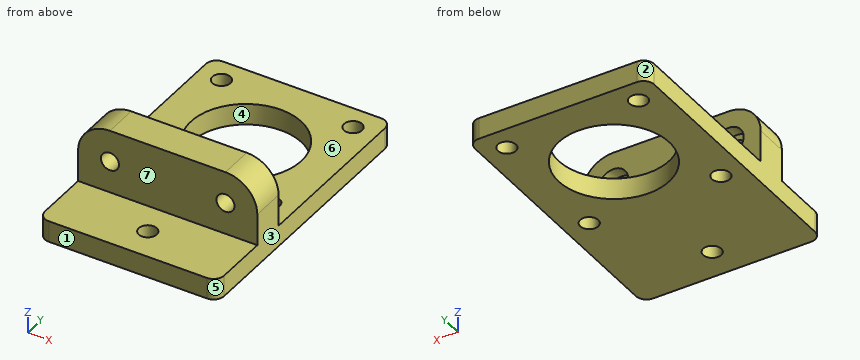
```python
from build123d import *

# Parameters (mm, degrees)
F0_R     = 2.125
F0_R_2   = 13
F1_DEPTH = 5
F2_W     = 42.2
F2_H     = 8
F3_DEPTH = 15
F4_R     = 7.5
F5_R     = 2.125
F6_DEPTH = 23.001
F7_R     = 3.5
F8_DEPTH = 3


with BuildPart() as f1:
    # F0 (on Top) → F1 (new body)
    with BuildSketch(Plane.XY):
        with BuildLine():
            Line((18.6, 21.1), (-18.6, 21.1))
            ThreePointArc((-18.6, 21.1), (-20.367767, 20.367767), (-21.1, 18.6))
            Line((-21.1, 18.6), (-21.1, -42))
            ThreePointArc((-21.1, -42), (-20.367767, -43.767767), (-18.6, -44.5))
            Line((-18.6, -44.5), (18.6, -44.5))
            ThreePointArc((18.6, -44.5), (20.367767, -43.767767), (21.1, -42))
            Line((21.1, -42), (21.1, 18.6))
            ThreePointArc((21.1, 18.6), (20.367767, 20.367767), (18.6, 21.1))
        make_face()
        with Locations((-15.5, -15.5)):
            Circle(F0_R, mode=Mode.SUBTRACT)
        with Locations((0, -37)):
            Circle(F0_R, mode=Mode.SUBTRACT)
        with Locations((15.5, -15.5)):
            Circle(F0_R, mode=Mode.SUBTRACT)
        with Locations((-15.5, 15.5)):
            Circle(F0_R, mode=Mode.SUBTRACT)
        Circle(F0_R_2, mode=Mode.SUBTRACT)
        with Locations((15.5, 15.5)):
            Circle(F0_R, mode=Mode.SUBTRACT)
    extrude(amount=F1_DEPTH)

    # F2 (on face) → F3 (join)
    with BuildSketch(Plane.XY.offset(5)):
        with Locations((0, -25.5)):
            Rectangle(F2_W, F2_H)
    extrude(amount=F3_DEPTH)

    # F4
    f4_edges = [f1.edges().sort_by_distance(p)[0] for p in [
        (-21.1, -25.5, 20),
        (21.1, -25.5, 20),
    ]]
    fillet(f4_edges, radius=F4_R)

    # F5 (on face) → F6 (cut, through all)
    with BuildSketch(Plane(origin=(0, -21.5, 0), x_dir=(-1, 0, 0), z_dir=(0, 1, 0))):
        with Locations((-13.6, 12.5)):
            Circle(F5_R)
        with Locations((13.6, 12.5)):
            Circle(F5_R)
    extrude(amount=-F6_DEPTH, mode=Mode.SUBTRACT)

    # F7 (on face) → F8 (cut)
    with BuildSketch(Plane(origin=(0, -21.5, 0), x_dir=(-1, 0, 0), z_dir=(0, 1, 0))):
        with Locations((-13.6, 12.5)):
            Circle(F7_R)
        with Locations((13.6, 12.5)):
            Circle(F7_R)
    extrude(amount=-F8_DEPTH, mode=Mode.SUBTRACT)


solid = f1.part
```
Work out the finished part from the listing and answer in its coordinate system (mm). Face numbers are marked on the shaded views. A direction names the side the tool comes from. Give positions to 0.01 mm unless a question says otherwise; leave off trailing zeros. Loops run counter-clockwise (first coordinate to the right, second up) from the corner with the lowest first, then second, coordinate; pieces in that order, holes last. Notation, with made-up numbers: M 53.25,-9.5 L 65.25,-9.5 A14 cw 65.25,13.5 Z; hole C -26,61.5 d7. An arc over 180 degrees is marked long. One line per item, written item: value. Start each with the question number.
1. Determine the mould class of the marked faces 1, 2, 3 and 4 for opening direction X: released by +X, released by -X, zero draft, split by the parting line, or undercut.
2. Find section B-B (y = -37). Give the vertices of the cut face in (x, z) (3 decimals), and give its area (3 significant figures).
3. Each of these flat-tipped pins is pushed along its axis until it touches: P1, Ø8, axis at x = 13.6, z = 12.5, coming from the -Y side; P2, Ø5, axis at x = 5, y = -13, coming from the +Z side; P3, Ø3.5, axis at x = -12, z = 12.5, coming from the +Y side; P4, Ø15.5, axis at x = 0, y = 0, coming from the +Z side. Where does it stop, or does it pass through?
4. Find the intervals of material crossed by probe 1 along X at (y, z) = (-25, 12.25); probe 2 along Y at (x, z) = (0, 2.4) (3 decimals); probe 3 along Y at (x, z) = (15.5, 1.8) (3 decimals), in increasing order.
5. Which of the six approach directions +Z, -Z, +X, -X, +Y, -Y give full straight-line access (tool end or side, diameter ignored) to the marked faces 5, 6 and 7?
6. Find section A-A (y = -15.5). Give the vertices of the cut face in (x, z) (3 decimals), and give its area (4 significant figures).
7. Find section D-D (x = -6). Give the vertices of the cut face in (y, z).
8. Find section C-C (x = 4.5). Give the vertices of the cut face in (y, z), and give its area (3 significant figures).
Reported:
1. face 1: zero draft
1. face 2: released by -X
1. face 3: released by +X
1. face 4: undercut
2. outline: M -21.1,0 L -2.125,0 L -2.125,5 L -21.1,5 Z; M 2.125,0 L 21.1,0 L 21.1,5 L 2.125,5 Z
2. area: 190 mm²
3. P1: stops at y = -29.5
3. P2: stops at z = 5
3. P3: stops at y = -24.5
3. P4: passes through
4. probe 1: x = -21.1 to -15.71, -11.49 to 11.49, 15.71 to 21.1
4. probe 2: y = -44.5 to -39.125, -34.875 to -13, 13 to 21.1
4. probe 3: y = -44.5 to -17.625, -13.375 to 13.375, 17.625 to 21.1
5. face 5: +Z, -Z, +X, -Y
5. face 6: +Z, +X, -X, +Y
5. face 7: +Z, +X, -X, -Y
6. outline: M -21.1,0 L -17.625,0 L -17.625,5 L -21.1,5 Z; M -13.375,0 L 13.375,0 L 13.375,5 L -13.375,5 Z; M 17.625,0 L 21.1,0 L 21.1,5 L 17.625,5 Z
6. area: 168.5 mm²
7. outline: M -44.5,0 L -11.53,0 L -11.53,5 L -21.5,5 L -21.5,20 L -29.5,20 L -29.5,5 L -44.5,5 Z; M 11.53,0 L 21.1,0 L 21.1,5 L 11.53,5 Z
8. outline: M -44.5,0 L -12.2,0 L -12.2,5 L -21.5,5 L -21.5,20 L -29.5,20 L -29.5,5 L -44.5,5 Z; M 12.2,0 L 21.1,0 L 21.1,5 L 12.2,5 Z
8. area: 326 mm²
